from build123d import *

# Parameters (mm, degrees)
EXTRUDE_1_DEPTH          = 2
HOLE_WIZARD_1_D          = 3.1
CUT_EXTRUDE_1_DEPTH      = 44
CUT_EXTRUDE_1_DEPTH_BACK = 44
SKETCH_5_W               = 102.055692614
SKETCH_5_H               = 55.211945292
CUT_EXTRUDE_2_DEPTH      = 44
CUT_EXTRUDE_2_DEPTH_BACK = 44


with BuildPart() as part:
    # 草图1 → 凸台-拉伸1 (new body)
    with BuildSketch(Plane(origin=(0, 0, 0), x_dir=(1, 0, 0), z_dir=(0, 1, 0))):
        with BuildLine():
            Line((35, 18), (-35, 18))
            ThreePointArc((-35, 18), (-37.828427125, 16.828427125), (-39, 14))
            Line((-39, 14), (-39, -14))
            ThreePointArc((-39, -14), (-37.828427125, -16.828427125), (-35, -18))
            Line((-35, -18), (35, -18))
            ThreePointArc((35, -18), (37.828427125, -16.828427125), (39, -14))
            Line((39, -14), (39, 14))
            ThreePointArc((39, 14), (37.828427125, 16.828427125), (35, 18))
        make_face()
    extrude(amount=EXTRUDE_1_DEPTH)

    # 孔1 (through all)
    with Locations(Plane(origin=(0, 2, 0), x_dir=(1, 0, 0), z_dir=(0, 1, 0))):
        with Locations((-8, 10), (-8, -10), (-35, -14), (-35, 14), (35, 14), (35, -14)):
            Hole(HOLE_WIZARD_1_D / 2)

    # 草图5 → 切除-拉伸1 (cut, two sides: drawn at the far end of the back side and taken through both)
    with BuildSketch(Plane(origin=(0, 2, 0), x_dir=(1, 0, 0), z_dir=(0, 1, 0)).offset(-CUT_EXTRUDE_1_DEPTH_BACK)):
        Rectangle(SKETCH_5_W, SKETCH_5_H)
        with BuildLine():
            Line((-11.560116303, 15.213061974), (-34.522933375, 17.971449035))
            ThreePointArc((-34.522933375, 17.971449035), (-37.65440516, 16.992345777), (-39, 14))
            Line((-39, 14), (-39, -14))
            ThreePointArc((-39, -14), (-37.65440516, -16.992345777), (-34.522933375, -17.971449035))
            Line((-34.522933375, -17.971449035), (-11.560116303, -15.213061974))
            ThreePointArc((-11.560116303, -15.213061974), (-8.714551025, -15.008553692), (-5.862458688, -15.076632276))
            Line((-5.862458688, -15.076632276), (34.713562836, -17.989731037))
            ThreePointArc((34.713562836, -17.989731037), (37.725275339, -16.927947118), (39, -14))
            Line((39, -14), (39, 14))
            ThreePointArc((39, 14), (37.725275339, 16.927947118), (34.713562836, 17.989731037))
            Line((34.713562836, 17.989731037), (-5.862458688, 15.076632276))
            ThreePointArc((-5.862458688, 15.076632276), (-8.714551025, 15.008553692), (-11.560116303, 15.213061974))
        make_face(mode=Mode.SUBTRACT)
    extrude(amount=CUT_EXTRUDE_1_DEPTH + CUT_EXTRUDE_1_DEPTH_BACK, mode=Mode.SUBTRACT)

    # 草图6 → 切除-拉伸2 (cut, two sides: drawn at the far end of the back side and taken through both)
    with BuildSketch(Plane(origin=(0, 2, 0), x_dir=(1, 0, 0), z_dir=(0, 1, 0)).offset(-CUT_EXTRUDE_2_DEPTH_BACK)):
        with BuildLine():
            Line((-2.125, 13.2), (29.5058803, 13.2))
            ThreePointArc((29.5058803, 13.2), (31.8808803, 10.825), (29.5058803, 8.45))
            Line((29.5058803, 8.45), (-2.125, 8.45))
            ThreePointArc((-2.125, 8.45), (-4.5, 10.825), (-2.125, 13.2))
        make_face()
        with BuildLine():
            Line((-13.875, 8.45), (-29.719593784, 8.45))
            ThreePointArc((-29.719593784, 8.45), (-32.094593784, 10.825), (-29.719593784, 13.2))
            Line((-29.719593784, 13.2), (-13.875, 13.2))
            ThreePointArc((-13.875, 13.2), (-11.5, 10.825), (-13.875, 8.45))
        make_face()
        with BuildLine():
            Line((-2.125, -13.2), (29.5058803, -13.2))
            ThreePointArc((29.5058803, -13.2), (31.8808803, -10.825), (29.5058803, -8.45))
            Line((29.5058803, -8.45), (-2.125, -8.45))
            ThreePointArc((-2.125, -8.45), (-4.5, -10.825), (-2.125, -13.2))
        make_face()
        with BuildLine():
            Line((-13.875, -8.45), (-29.719593784, -8.45))
            ThreePointArc((-29.719593784, -8.45), (-32.094593784, -10.825), (-29.719593784, -13.2))
            Line((-29.719593784, -13.2), (-13.875, -13.2))
            ThreePointArc((-13.875, -13.2), (-11.5, -10.825), (-13.875, -8.45))
        make_face()
        with BuildLine():
            Line((-31.05, 5.45), (-14.7, 5.45))
            ThreePointArc((-14.7, 5.45), (-9.25, 0), (-14.7, -5.45))
            Line((-14.7, -5.45), (-31.05, -5.45))
            ThreePointArc((-31.05, -5.45), (-36.5, 0), (-31.05, 5.45))
        make_face()
        with BuildLine():
            Line((-1.3, 5.45), (31.05, 5.45))
            ThreePointArc((31.05, 5.45), (36.5, 0), (31.05, -5.45))
            Line((31.05, -5.45), (-1.3, -5.45))
            ThreePointArc((-1.3, -5.45), (-6.75, 0), (-1.3, 5.45))
        make_face()
    extrude(amount=CUT_EXTRUDE_2_DEPTH + CUT_EXTRUDE_2_DEPTH_BACK, mode=Mode.SUBTRACT)


solid = part.part
The listing builds one solid part. Answer for the finished solid, in the listing's coordinates (mm). A direction names the side the tool comes from. Coordinates: 2 decimals unless noted, no trailing zeros. Order: outer loops, then holes, each group sorted by start corner. A loop starts at its lowest first (then second) coordinate and runs counter-clockwise, first axis right, second up. Notation, with made-up numbers: (-39.75, 47.25) -> (-26.75, 47.25) arc R19 ccw to (-26.75, 70.25) -> close; hole circle Ø4 at (38.25, -7). An arc over 180 degrees is marked (long way). Answer in a Markdown table with one row per item. Add a question column.
Item 1: Determine the mould class of faces 1 (the face through (13, 1, -13.2)), 2 (the face through (-9, 2, 0)), 3 (the face through (-39, 1, 0)) for opening direction X: +X half, -X half, draft (parallel to the pull), parting line (faces both ways), or undercut.
Item 2: Find section B-B (x = -8). Write down the section's boundary in (y, z), then the cut area to 3 significant figures.
Item 3: Each of these flat-tipped pins is pushed along its axis until it touches: P1, Ø0.6, axis at x = -22, y = 1.5, coming from the -Z side; P2, Ø0.6, axis at x = -24, y = 1, coming from the +Z side; P3, Ø0.6, axis at x = 11, y = 1, coming from the +Z side. Where does it stop, or does it pass through?
Item 4: Find section C-C (x = 12.5). Write down the section's boundary in (y, z), then the cut area to 3 significant figures.
Item 5: Find section A-A (z = 3). Write down the section's boundary in (x, y).
Item 6: Find the intervals of material crossed by L1, parallel to X at y = 0.65, z = -14; L2, parallel to Z at x = 0.5, y = 1.65; L3, parallel to X at y = 1.55, z = 10, in increasing order. Write a range as from..to.
Item 7: Which of the six approach directions +Z, -Z, +X, -X, +Y, -Y give full straight-line access (tool end or side, diameter ignored) to faces 4 (the face through (13, 1, 13.2)), 5 (the face through (-23.2, 0.99, 16.61)), 6 (the face through (-8.675, 0.986, -15.008))?
Item 8: Find section D-D (y = 1). State how many separate pieces and enclosed holes the cut face has, then the cut area to 3 significant figures.
Result set:
| question | item | result |
|---|---|---|
| 1 | face 1 | undercut |
| 1 | face 2 | draft |
| 1 | face 3 | -X half |
| 2 | outline | (0, -15) -> (2, -15) -> (2, -11.55) -> (0, -11.55) -> close; (0, -8.45) -> (2, -8.45) -> (2, 8.45) -> (0, 8.45) -> close; (0, 11.55) -> (2, 11.55) -> (2, 15) -> (0, 15) -> close |
| 2 | area | 47.6 mm² |
| 3 | P1 | stops at z = -16.5 |
| 3 | P2 | stops at z = 16.74 |
| 3 | P3 | stops at z = 16.31 |
| 4 | outline | (0, -16.39) -> (2, -16.39) -> (2, -13.2) -> (0, -13.2) -> close; (0, -8.45) -> (2, -8.45) -> (2, -5.45) -> (0, -5.45) -> close; (0, 5.45) -> (2, 5.45) -> (2, 8.45) -> (0, 8.45) -> close; (0, 13.2) -> (2, 13.2) -> (2, 16.39) -> (0, 16.39) -> close |
| 4 | area | 24.8 mm² |
| 5 | outline | (-39, 0) -> (-35.6, 0) -> (-35.6, 2) -> (-39, 2) -> close; (-10.15, 0) -> (-5.85, 0) -> (-5.85, 2) -> (-10.15, 2) -> close; (35.6, 0) -> (39, 0) -> (39, 2) -> (35.6, 2) -> close |
| 6 | L1 | x = -39..-36.55, -33.45..33.45, 36.55..39 |
| 6 | L2 | z = -15.53..-13.2, -8.45..-5.45, 5.45..8.45, 13.2..15.53 |
| 6 | L3 | x = -39..-31.95, -11.65..-9.55, -6.45..-4.35, 31.73..39 |
| 7 | face 4 | +Y, -Y |
| 7 | face 5 | +Z, +Y, -Y |
| 7 | face 6 | -Z, +Y, -Y |
| 8 | separate pieces | 1 |
| 8 | enclosed holes | 12 |
| 8 | area | 1,290 mm² |
